```python
from build123d import *

# Parameters (mm, degrees)
SKETCH_1_W          = 34.967301983
SKETCH_1_H          = 16.2
EXTRUDE_1_DEPTH     = 0.5
EXTRUDE_START       = -1.7
EXTRUDE_2_DEPTH     = 1.7
SKETCH_2_R          = 0.950019994
SKETCH_2_R_2        = 0.963923892
SKETCH_2_R_3        = 0.95
CUT_EXTRUDE_4_DEPTH = 27.925670861


with BuildPart() as part:
    # Sketch 1 → Extrude 1 (new body)
    # profile 1 of 3: a face of its own
    with BuildSketch(Plane(origin=(0, 0, 0), x_dir=(1, 0, 0), z_dir=(0, 1, 0))):
        Polygon((22.288172203, 7.655913898), (22.288172203, 7.855913898), (22.288172203, 9.255913898), (20.988172203, 10.555913898), (-23.011827797, 10.555913898), (-24.711827797, 8.855913898), (-24.711827797, -8.344086102), (-23.011827797, -10.044086102), (19.388172203, -10.044086102), (22.288172203, -7.144086102), (22.288172203, -3.344086102), (22.288172203, -3.144086102), (21.901185097, -3.144086102), (19.928457532, -4.644944449), (19.928457532, -5.544086102), (19.028457532, -5.544086102), (19.028457532, -4.544086102), (16.255474186, -4.544086102), (16.255474186, -8.444086102), (-19.911827797, -8.444086102), (-19.911827797, -6.744086102), (-20.711827797, -5.944086102), (-20.711827797, 6.455913898), (-19.911827797, 7.255913898), (-19.911827797, 8.955913898), (16.255474186, 8.955913898), (16.255474186, 8.258604903), (18.488172203, 7.888602523), (18.488172203, 8.855913898), (20.432236612, 8.855913898), (21.931117854, 7.655913898), align=None)
    # profile 2 of 3: a face of its own
    with BuildSketch(Plane(origin=(0, 0, 0), x_dir=(1, 0, 0), z_dir=(0, 1, 0))):
        with BuildLine():
            Line((22.288172203, 6.587195464), (22.288172203, 7.655913898))
            Line((22.288172203, 7.655913898), (21.931117854, 7.655913898))
            Line((21.931117854, 7.655913898), (20.432236612, 8.855913898))
            Line((20.432236612, 8.855913898), (18.488172203, 8.855913898))
            Line((18.488172203, 8.855913898), (18.488172203, 7.888602523))
            Line((18.488172203, 7.888602523), (16.255474186, 8.258604903))
            Line((16.255474186, 8.258604903), (16.255474186, -4.544086102))
            Line((16.255474186, -4.544086102), (19.028457532, -4.544086102))
            Line((19.028457532, -4.544086102), (19.028457532, -5.544086102))
            Line((19.028457532, -5.544086102), (19.928457532, -5.544086102))
            Line((19.928457532, -5.544086102), (19.928457532, -4.644944449))
            Line((19.928457532, -4.644944449), (21.901185097, -3.144086102))
            Line((21.901185097, -3.144086102), (22.288172203, -3.144086102))
            Line((22.288172203, -3.144086102), (22.288172203, -2.075367667))
            ThreePointArc((22.288172203, -2.075367667), (23.688172203, 2.255913898), (22.288172203, 6.587195464))
        make_face()
    # profile 3 of 3: a face of its own
    with BuildSketch(Plane(origin=(0, 0, 0), x_dir=(1, 0, 0), z_dir=(0, 1, 0))):
        Polygon((-20.711827797, 6.455913898), (-19.911827797, 7.255913898), (-19.911827797, 8.955913898), (16.255474186, 8.955913898), (16.255474186, -8.444086102), (-19.911827797, -8.444086102), (-19.911827797, -6.744086102), (-20.711827797, -5.944086102), align=None)
        with Locations((-1.828176806, 0.255913898)):
            Rectangle(SKETCH_1_W, SKETCH_1_H, mode=Mode.SUBTRACT)
    extrude(amount=EXTRUDE_1_DEPTH)

    # Sketch 1_3 → Extrude 2 (add)
    with BuildSketch(Plane(origin=(0, 0, 0), x_dir=(1, 0, 0), z_dir=(0, 1, 0)).offset(EXTRUDE_START)):
        with BuildLine():
            Line((22.288172203, 6.587195464), (22.288172203, 7.655913898))
            Line((22.288172203, 7.655913898), (21.931117854, 7.655913898))
            Line((21.931117854, 7.655913898), (20.432236612, 8.855913898))
            Line((20.432236612, 8.855913898), (18.488172203, 8.855913898))
            Line((18.488172203, 8.855913898), (18.488172203, 7.888602523))
            Line((18.488172203, 7.888602523), (16.255474186, 8.258604903))
            Line((16.255474186, 8.258604903), (16.255474186, -4.544086102))
            Line((16.255474186, -4.544086102), (19.028457532, -4.544086102))
            Line((19.028457532, -4.544086102), (19.028457532, -5.544086102))
            Line((19.028457532, -5.544086102), (19.928457532, -5.544086102))
            Line((19.928457532, -5.544086102), (19.928457532, -4.644944449))
            Line((19.928457532, -4.644944449), (21.901185097, -3.144086102))
            Line((21.901185097, -3.144086102), (22.288172203, -3.144086102))
            Line((22.288172203, -3.144086102), (22.288172203, -2.075367667))
            ThreePointArc((22.288172203, -2.075367667), (23.688172203, 2.255913898), (22.288172203, 6.587195464))
        make_face()
    extrude(amount=EXTRUDE_2_DEPTH)

    # Sketch 2 → Cut-Extrude 4 (cut, through all)
    with BuildSketch(Plane(origin=(0, 0, 0), x_dir=(1, 0, 0), z_dir=(0, 1, 0))):
        with Locations(Location((-22.111827797, 8.255913898, 0), (0, 0, 270))):
            Circle(SKETCH_2_R)
        with Locations(Location((-22.123719351, -7.736880442, 0), (0, 0, 270))):
            Circle(SKETCH_2_R_2)
        with Locations(Location((18.488191089, -7.744092667, 0), (0, 0, 270))):
            Circle(SKETCH_2_R_3)
    extrude(amount=CUT_EXTRUDE_4_DEPTH, mode=Mode.SUBTRACT)


solid = part.part
```
Check sheet for the modelled part. Datum: model origin and axes. Units: mm. A direction names the side the tool comes from. Give positions to 0.01 mm unless a question says otherwise; leave off trailing zeros. Loops run counter-clockwise (first coordinate to the right, second up) from the corner with the lowest first, then second, coordinate; pieces in that order, holes last. Notation, with made-up numbers: (-15.75, -14.5) - (7.25, -14.5) arc R10 ccw to (7.25, -9.5) - close; hole circle Ø8 at (-23.75, 48.5). An arc over 180 degrees is marked (long way). One line per question, with ' | ' between items. Start each with the question number.
1. Cross-section at A-A, the plane x = 8. Enter the section's corners in (y, z), plus the area to 3 significant figures.
2. Material ranges on line 1 along Y through (x, z) = (-20, 5); line 2 along X through (y, z) = (-0.05, -6.75); line 3 along X through (y, z) = (0.05, -5.75), recorded low to high. Write a range as [from, to].
3. Cross-section at D-D, the plane z = -1.75. Enter the section's corners in (x, y), plus the area to 3 significant figures.
4. Cross-section at C-C, the plane y = -0.4. Enter the section's corners in (x, z).
5. Set-up check for faces 1 (the flat face through (18.488, -0.9, -8.4)), 2 (the flat face through (16.255, -1, -2)), 3 (the flat face through (22.288, -0.13, 2.96)): record each of +Z, -Z, +X, -X, +Y, -Y from which the full face is reachable in a straight line by a thin tool's end or side.
6. Draft check along X on faces 4 (the cylindrical face through (19.43, 0.25, 7.62)), 5 (the flat face through (18, -1, 4.544)), 6 (the flat face through (21.19, -0.86, -8.25)). Enter one of: released by +X, released by -X, zero draft, split by the parting line, or undercut.
7. Cross-section at B-B, the plane z = -4.5. Enter the section's corners in (x, y).
8. Gauge pin test, flat ends, axial feed: pin 1 Ø0.5 at (y, z) = (-0.5, -1) entering from -X; pin 2 Ø0.5 at (y, z) = (-1, 5) entering from -X; pin 3 Ø0.8 at (x, y) = (19, -0.5) entering from -Z; pin 4 Ø2 at (x, z) = (18.49, 7.74) entering from +Y. Record the tip position at first contact, or that the pin passes through.
Check result:
1) outline: (0, -10.56) - (0.5, -10.56) - (0.5, -8.36) - (0, -8.36) - close; (0, 7.84) - (0.5, 7.84) - (0.5, 10.04) - (0, 10.04) - close | area: 2.20 mm2
2) line 1: y = [0, 0.5] | line 2: x = [16.26, 22.29] | line 3: x = [-24.71, -19.31], [15.66, 22.81]
3) outline: (-24.71, 0) - (-19.31, 0) - (-19.31, 0.5) - (-24.71, 0.5) - close; (15.66, 0) - (16.26, 0) - (16.26, -1.7) - (23.67, -1.7) - (23.67, 0.5) - (15.66, 0.5) - close | area: 19.3 mm2
4) outline: (16.26, -8.26) - (18.49, -7.89) - (18.49, -8.86) - (20.43, -8.86) - (21.93, -7.66) - (22.29, -7.66) - (22.29, -6.59) arc R7.4 ccw to (22.29, 2.08) - (22.29, 3.14) - (21.9, 3.14) - (19.93, 4.64) - (19.93, 5.54) - (19.03, 5.54) - (19.03, 4.54) - (16.26, 4.54) - close
5) face 1: -Z, -Y | face 2: +Z, -Z, -X, -Y | face 3: +Z, +X, +Y, -Y
6) face 4: undercut | face 5: zero draft | face 6: released by +X
7) outline: (-24.71, 0) - (-19.31, 0) - (-19.31, 0.5) - (-24.71, 0.5) - close; (15.66, 0) - (16.26, 0) - (16.26, -1.7) - (23.34, -1.7) - (23.34, 0.5) - (15.66, 0.5) - close
8) pin 1: stops at x = 16.26 | pin 2: stops at x = 19.03 | pin 3: stops at z = -8.86 | pin 4: stops at y = 0.5
